Job drawing, mm, ordinate dimensions from the low corner. One solid piece. A direction names the side the tool comes from. Give positions to 0.01 mm unless a question says otherwise; leave off trailing zeros. Order: outer loops, then holes, each group sorted by start corner. A loop starts at its lowest first (then second) coordinate and runs counter-clockwise, first axis right, second up. Notation, with made-up numbers: (19, -25) - (31, -25) arc R14 ccw to (31, -21) - close; hole circle Ø2 at (57, -26.75). An arc over 180 degrees is marked (long way). Use one line per item in the form item = value. Start each with the question number.
1. Band-saw the part on C-C, the plane z = 5.5. List the corners of the cut face in (x, y), plus the area to 3 significant figures.
2. Pull direction X, two halves, no side cores. Call the marked faces 6, 7, 8 and 9: +X half, -X half, draft (parallel to the pull), parting line (faces both ways), or undercut.
3. Drill centre lines: line 1 (Y direction, x = 10, z = 11.75); line 2 (X direction, y = 7.8, z = 11); line 3 (Y direction, x = 10, z = 0.95). Where is each one in solid material? Low to high.
4. Band-saw the part on B-B, the plane y = 7.8. List the corners of the cut face in (x, z), plus the area to 3 significant figures.
5. Band-saw the part on D-D, the plane y = 14. List the corners of the cut face in (x, z), plus the area to 3 significant figures.
6. Band-saw the part on A-A, the plane x = 10. List the corners of the cut face in (y, z).
7. Pin check, flat tips, straight feed: P1, Ø1, axis at x = 17.5, z = 2.5, coming from the +Y side; P2, Ø3.5, axis at x = 17.5, z = 2.5, coming from the -Y side; P3, Ø4, axis at x = 8, z = 3, coming from the +Y side. Stop position of each tip, or through.
8. Tool access for the marked faces 1, 2, 3, 4 and 5: list every direction of +Z, -Z, +X, -X, +Y, -Y with a clear straight run to the whole face (end or side of a thin tool).
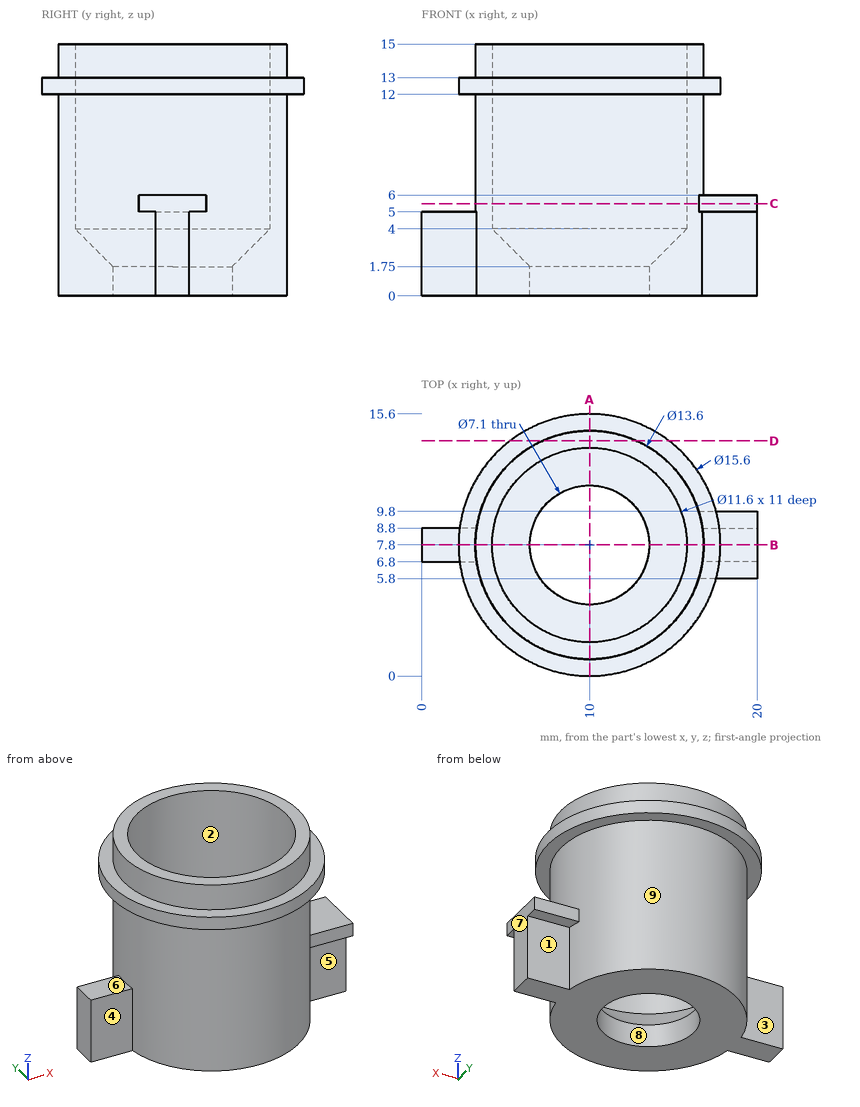
From the geometry:
q1.outline = (16.5, 5.8) - (20, 5.8) - (20, 9.8) - (16.5, 9.8) arc R6.8 ccw (long way) to start; hole circle Ø11.6 at (10, 7.8)
q1.area = 52.8 mm²
q2.face_6 = draft
q2.face_7 = +X half
q2.face_8 = undercut
q2.face_9 = parting line
q3.line_1 = 1 to 2, 13.6 to 14.6
q3.line_2 = 3.2 to 4.2, 15.8 to 16.8
q3.line_3 = 1 to 4.25, 11.35 to 14.6
q4.outline = (0, 0) - (6.45, 0) - (6.45, 1.75) - (4.2, 4) - (4.2, 15) - (3.2, 15) - (3.2, 13) - (2.2, 13) - (2.2, 12) - (3.2, 12) - (3.2, 5) - (0, 5) - close; (13.55, 0) - (20, 0) - (20, 6) - (16.8, 6) - (16.8, 12) - (17.8, 12) - (17.8, 13) - (16.8, 13) - (16.8, 15) - (15.8, 15) - (15.8, 4) - (13.55, 1.75) - close
q4.area = 80.1 mm²
q5.outline = (5.27, 12) - (7.21, 12) - (7.21, 0) - (12.79, 0) - (12.79, 12) - (14.73, 12) - (14.73, 13) - (12.79, 13) - (12.79, 15) - (7.21, 15) - (7.21, 13) - (5.27, 13) - close
q5.area = 87.7 mm²
q6.outline = (0, 12) - (1, 12) - (1, 0) - (4.25, 0) - (4.25, 1.75) - (2, 4) - (2, 15) - (1, 15) - (1, 13) - (0, 13) - close; (11.35, 0) - (14.6, 0) - (14.6, 12) - (15.6, 12) - (15.6, 13) - (14.6, 13) - (14.6, 15) - (13.6, 15) - (13.6, 4) - (11.35, 1.75) - close
q7.P1 = 8.8
q7.P2 = 4.17
q7.P3 = 14.6
q8.face_1 = -Z, +X, +Y
q8.face_2 = +Z
q8.face_3 = -Z, -X, +Y
q8.face_4 = -Z, -X, -Y
q8.face_5 = -Z, +X, -Y
